For this review, take the finished solid that the model builds, in its own axes (mm). A direction names the side the tool comes from. Give positions to 0.01 mm unless a question says otherwise; leave off trailing zeros. Loops run counter-clockwise (first coordinate to the right, second up) from the corner with the lowest first, then second, coordinate; pieces in that order, holes last.
Autodesk Inventor part; units mm, degrees
ref_plane "YZ Plane" through (0, 0, 0) normal (1, 0, 0) x (0, 1, 0)
ref_plane "XZ Plane" through (0, 0, 0) normal (0, 1, 0) x (-1, 0, 0)
ref_plane "XY Plane" through (0, 0, 0) normal (0, 0, 1) x (1, 0, 0)
sketch "Skizze1" plane through (0, 0, 0) normal (0, 0, 1) x (1, 0, 0)
  line L0 (-2.6992, -1.5246) -> (2.6992, -1.5246)
  circle A0 centre (0, 0) radius 6
  arc A1 (2.6992, -1.5246) -> (-2.6992, -1.5246) centre (0, 0) ccw
  dimension "d3" = 12
  dimension "d6" = 6.2
extrude "Extrusion1" add sketch "Skizze1" along normal blind 11
sketch "Skizze4" plane through (0, 0, 11) normal (0, 0, 1) x (1, 0, 0)
  circle A0 centre (0, 0) radius 6
  dimension "d14" = 12
extrude "Extrusion3" add sketch "Skizze4" along normal blind 2
sketch "Skizze5" plane through (0, 0, 13) normal (0, 0, 1) x (1, 0, 0)
  line L0 (-2.45, 4.95) -> (2.45, 4.95)
  line L1 (2.45, 4.95) -> (2.45, -4.95)
  line L2 (2.45, -4.95) -> (-2.45, -4.95)
  line L3 (-2.45, -4.95) -> (-2.45, 4.95)
  point P0 (0, 0)
  point P1 (0, 0)
  dimension "d17" = 4.9
  dimension "d18" = 9.9
  dimension "d19" = 2.45
  dimension "d20" = 4.95
extrude "Extrusion4" add sketch "Skizze5" along normal blind 9
properties part number "AdapterPoti2"
Q1. Consider section C-C on z = 7. Give the boundary of the cut face in (x, y), plus the area to 3 significant figures.
Answers:
outline: circle Ø12 at (0, 0); hole (-2.7, -1.52) - (2.7, -1.52) arc R3.1 ccw (long way) to start
area: 88.9 mm2
Q2. For probe 1 along Y at (x, z) = (0, 2.5); probe 2 along X at (y, z) = (-0.5, 14); probe 3 along Z at (x, y) = (-3.5, -1), list the stretches that pass through material, from the lowest coordinate up.
Answers:
probe 1: y = -6 to -1.52, 3.1 to 6
probe 2: x = -2.45 to 2.45
probe 3: z = 0 to 13
Q3. Consider section B-B on x = 0. Give the boundary of the cut face in (y, z), plus the area to 3 significant figures.
Answers:
outline: (-6, 0) - (-1.52, 0) - (-1.52, 11) - (3.1, 11) - (3.1, 0) - (6, 0) - (6, 13) - (4.95, 13) - (4.95, 22) - (-4.95, 22) - (-4.95, 13) - (-6, 13) - close
area: 194 mm2
Q4. Consider section A-A on y = 0. Give the boundary of the cut face in (x, z).
Answers:
outline: (-6, 0) - (-3.1, 0) - (-3.1, 11) - (3.1, 11) - (3.1, 0) - (6, 0) - (6, 13) - (2.45, 13) - (2.45, 22) - (-2.45, 22) - (-2.45, 13) - (-6, 13) - close
Q5. For pin 1 Ø5 at (y, z) = (3, 8.5) entering from -X; pin 2 Ø1.4 at (x, y) = (-1, 0.5) entering from -Z; pin 3 Ø7 at (y, z) = (-1.5, 18) entering from -X, all flat-tipped, find the tip position at first contact; note any pin that passes through.
Answers:
pin 1: stops at x = -5.98
pin 2: stops at z = 11
pin 3: stops at x = -2.45
Q6. Mouldability with a two-part tool opening along X and no side actions: class faces 1 (the cylindrical face through (-6, 0, 6)), 2 (the cylindrical face through (-0.1, 3.1, 5.4)), 3 (the flat face through (-2.45, 0, 17)), 4 (the flat face through (0, -4.95, 17)) as +X half, -X half, draft (parallel to the pull), parting line (faces both ways), or undercut.
Answers:
face 1: parting line
face 2: undercut
face 3: -X half
face 4: draft
Q7. Consider section D-D on z = 12.25. Give the boundary of the cut face in (x, y), plus the area to 3 significant figures.
Answers:
outline: circle Ø12 at (0, 0)
area: 113 mm2
Q8. Machinability: for faces 5 (the flat face through (0, 0, 22)), 6 (the flat face through (0, 4.95, 17)), 7 (the flat face through (2.45, 0, 17)), 8 (the flat face through (0, 0, 11)), which of the approach directions +Z, -Z, +X, -X, +Y, -Y give a long, thin tool a straight path to every point of the face, cutting with its end or side? Answer none if there is none.
Answers:
face 5: +Z, +X, -X, +Y, -Y
face 6: +Z, +X, -X, +Y
face 7: +Z, +X, +Y, -Y
face 8: -Z
